For this review, use the dimensioned drawing (mm, ordinates from the lowest corner) and the shaded views. A direction names the side the tool comes from. Coordinates: 2 decimals unless noted, no trailing zeros. Order: outer loops, then holes, each group sorted by start corner. A loop starts at its lowest first (then second) coordinate and runs counter-clockwise, first axis right, second up. Notation, with made-up numbers: M 74.5,-38.75 L 98.5,-38.75 A19 cw 98.5,-7.75 Z; hole C 80.5,-36.5 d1. An arc over 180 degrees is marked long. Answer in a Markdown table with one row per item.
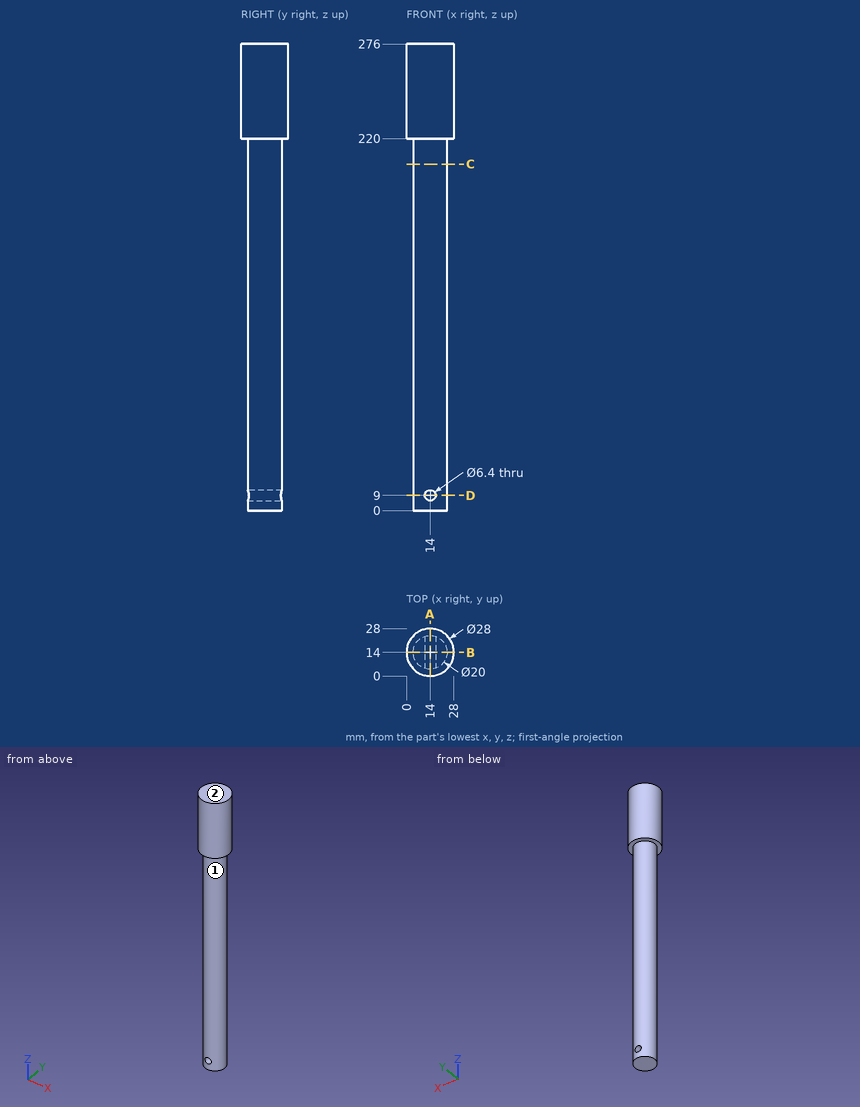
(1) For the marked faces 1 and 2, list the 3-axis set-ups (+Z, -Z, +X, -X, +Y, -Y) from which the entire face can be reached by the end or side of a thin tool; tool diameter is ignored.
Return value:
| item | result |
|---|---|
| face 1 | -Z |
| face 2 | +Z, +X, -X, +Y, -Y |
(2) Insertion check: pin 1 Ø4 at (x, z) = (8.5, 245) entering from +Y; pin 2 Ø3 at (x, z) = (8, 72.5) entering from +Y; pin 3 Ø5 at (y, z) = (9.5, 102.5) entering from +X. Each pin has a flat end and moves straight along its axis. Give the tip position at first contact, or say it passes through.
Return value:
| item | result |
|---|---|
| pin 1 | stops at y = 27.56 |
| pin 2 | stops at y = 22.93 |
| pin 3 | stops at x = 23.8 |
(3) Add section D-D, the plane z = 9. Give the boundary of the cut face in (x, y).
Return value:
| item | result |
|---|---|
| outline | M 10.8,4.53 L 10.8,23.47 A10 ccw Z; M 17.2,4.53 A10 ccw 17.2,23.47 Z |
(4) Add section B-B, the plane y = 14. Give the boundary of the cut face in (x, z), and give its area (3 significant figures).
Return value:
| item | result |
|---|---|
| outline | M 0,220 L 4,220 L 4,0 L 24,0 L 24,220 L 28,220 L 28,276 L 0,276 Z; hole C 14,9 d6.4 |
| area | 5,940 mm2 |
(5) Add section A-A, the plane x = 14. Give the boundary of the cut face in (y, z), and give its area (3 significant figures).
Return value:
| item | result |
|---|---|
| outline | M 0,220 L 4,220 L 4,12.2 L 24,12.2 L 24,220 L 28,220 L 28,276 L 0,276 Z; M 4,0 L 24,0 L 24,5.8 L 4,5.8 Z |
| area | 5,840 mm2 |
(6) For line 1 along Z through (x, y) = (14, 17.25); line 2 along Z through (x, y) = (24.75, 16.5); line 3 along Z through (x, y) = (12.5, 23), list the stretches that pass through material, from the lowest coordinate up. Write a range as from..to.
Return value:
| item | result |
|---|---|
| line 1 | z = 0..5.8, 12.2..276 |
| line 2 | z = 220..276 |
| line 3 | z = 0..6.17, 11.83..276 |
(7) Add section C-C, the plane z = 205. Give the boundary of the cut face in (x, y), and give its area (3 significant figures).
Return value:
| item | result |
|---|---|
| outline | C 14,14 d20 |
| area | 314 mm2 |
